from build123d import *

# Parameters (mm, degrees)
F0_R     = 25
F0_R_2   = 2.5
F0_R_3   = 4
F1_DEPTH = 6
F2_R     = 12.5
F2_R_2   = 4
F3_DEPTH = 30
F4_SIZE  = 1


with BuildPart() as f1:
    # F0 (on Top) → F1 (new body)
    with BuildSketch(Plane.XY):
        Circle(F0_R)
        with Locations((-20, 0)):
            Circle(F0_R_2, mode=Mode.SUBTRACT)
        Circle(F0_R_3, mode=Mode.SUBTRACT)
        with Locations((20, 0)):
            Circle(F0_R_2, mode=Mode.SUBTRACT)
    extrude(amount=F1_DEPTH)

    # F2 (on face) → F3 (join)
    with BuildSketch(Plane.XY.offset(6)):
        Circle(F2_R)
        Circle(F2_R_2, mode=Mode.SUBTRACT)
    extrude(amount=F3_DEPTH)

    # F4
    f4_edges = [f1.edges().sort_by_distance(p)[0] for p in [
        (-12.5, 0, 36),
        (-25, 0, 6),
        (-25, 0, 0),
    ]]
    chamfer(f4_edges, length=F4_SIZE)


solid = f1.part
Geometry: final body of the model. Coordinates: model frame, mm. A direction names the side the tool comes from. Coordinates: 2 decimals unless noted, no trailing zeros. Order: outer loops, then holes, each group sorted by start corner. A loop starts at its lowest first (then second) coordinate and runs counter-clockwise, first axis right, second up.
1) Section B-B (x = 0). Return loops of the section in (y, z).
Result sheet:
outline: (-25, 1) - (-24, 0) - (-4, 0) - (-4, 36) - (-11.5, 36) - (-12.5, 35) - (-12.5, 6) - (-24, 6) - (-25, 5) - close; (4, 0) - (24, 0) - (25, 1) - (25, 5) - (24, 6) - (12.5, 6) - (12.5, 35) - (11.5, 36) - (4, 36) - close
2) Section C-C (z = 14). Return loops of the section in (x, y), then the cut area to 3 significant figures.
Result sheet:
outline: circle Ø25 at (0, 0); hole circle Ø8 at (0, 0)
area: 441 mm2
3) Ray query, probe 1 along Y at (x, z) = (0, 26.5); probe 2 along Y at (x, z) = (-3.5, 18.5); probe 3 along Z at (x, y) = (7.5, 16). Return the intervals inside material, ascending.
Result sheet:
probe 1: y = -12.5 to -4, 4 to 12.5
probe 2: y = -12 to -1.94, 1.94 to 12
probe 3: z = 0 to 6
4) Set-up query: faces 1 (the flat face through (5, 0, 0)), 2 (the cylindrical face through (11.923, 3.755, 20.297)). Return all of +Z, -Z, +X, -X, +Y, -Y with unobstructed straight access to the full face (end or side cutting, diameter ignored); none if empty.
Result sheet:
face 1: -Z, +X, -X, +Y, -Y
face 2: +Z
5) Section A-A (y = 0). Return loops of the section in (x, z), then the cut area to 3 significant figures.
Result sheet:
outline: (-25, 1) - (-24, 0) - (-22.5, 0) - (-22.5, 6) - (-24, 6) - (-25, 5) - close; (-17.5, 0) - (-4, 0) - (-4, 36) - (-11.5, 36) - (-12.5, 35) - (-12.5, 6) - (-17.5, 6) - close; (4, 0) - (17.5, 0) - (17.5, 6) - (12.5, 6) - (12.5, 35) - (11.5, 36) - (4, 36) - close; (22.5, 0) - (24, 0) - (25, 1) - (25, 5) - (24, 6) - (22.5, 6) - close
area: 699 mm2
6) First-contact query: P1, Ø5, axis at y = 9, z = 15.5, coming from the -X side; P2, Ø4, axis at y = -8, z = 26, coming from the +X side; P3, Ø1, axis at x = 11, y = -5, coming from the +Z side; P4, Ø4, axis at x = -20, y = 0, coming from the +Z side. Flat tips, straight axial feed; report the tip coordinate or a pass-through.
Result sheet:
P1: stops at x = -10.68
P2: stops at x = 10.97
P3: stops at z = 35.92
P4: passes through
7) Draft query along Y for faces 3 (the flat face through (5, 0, 36)), 4 (the cylindrical face through (-22.5, 0.1, 3)), 5 (the cylindrical face through (17.5, 0.1, 3)), 6 (the cylindrical face through (23.846, 7.509, 2.972)). Return one class per face: released by +Y, released by -Y, zero draft, split by the parting line, or undercut.
Result sheet:
face 3: zero draft
face 4: undercut
face 5: undercut
face 6: split by the parting line
